Autodesk Inventor part; units mm, degrees
ref_plane "YZ Plane" through (0, 0, 0) normal (1, 0, 0) x (0, 1, 0)
ref_plane "XZ Plane" through (0, 0, 0) normal (0, 1, 0) x (-1, 0, 0)
ref_plane "XY Plane" through (0, 0, 0) normal (0, 0, 1) x (1, 0, 0)
sketch "Sketch1" plane through (0, 0, 0) normal (0, 1, 0) x (-1, 0, 0)
  line L0 (32, 32) -> (0, 32)
  line L1 (0, 32) -> (0, 0)
  line L2 (0, 0) -> (32, 0)
  line L3 (32, 0) -> (32, 32)
extrude "Extrusion1" add sketch "Sketch1" along normal blind 55
sketch "Sketch2" plane through (0, 55, 0) normal (0, 1, 0) x (1, 0, 0)
  line L0 (-9.6, -9.6) -> (-22.4, -9.6)
  line L1 (-22.4, -9.6) -> (-22.4, -22.4)
  line L2 (-22.4, -22.4) -> (-9.6, -22.4)
  line L3 (-9.6, -22.4) -> (-9.6, -9.6)
  point P0 (0, 0)
extrude "Extrusion2" cut sketch "Sketch2" against normal blind 30
sketch "Sketch3" plane through (-32, 0, 32) normal (0, 0, 1) x (1, 0, 0)
  line L0 (3.5, 49) -> (28.5, 49)
  line L1 (28.5, 49) -> (28.5, 31)
  line L2 (28.5, 31) -> (3.5, 31)
  line L3 (3.5, 31) -> (3.5, 49)
  line L4 (3.5, 49) -> (3.5, 43.25)
  line L5 (3.5, 36.75) -> (3.5, 43.25)
  line L6 (28.5, 49) -> (28.5, 43.25)
  line L7 (28.5, 36.75) -> (28.5, 43.25)
  line L8 (3.5, 43.25) -> (3.5, 36.75)
  line L9 (28.5, 43.25) -> (28.5, 36.75)
  point P0 (32, 0)
extrude "Extrusion3" cut sketch "Sketch3" against normal blind 2.5
sketch "Sketch4" plane through (-32, 0, 29.5) normal (0, 0, 1) x (1, 0, 0)
  line L0 (3.5, 49) -> (28.5, 49)
  line L1 (3.5, 49) -> (3.5, 43.25)
  line L2 (28.5, 31) -> (3.5, 31)
  line L3 (3.5, 36.75) -> (3.5, 31)
  line L4 (3.5, 31) -> (28.5, 31)
  line L5 (28.5, 31) -> (28.5, 36.75)
  line L6 (28.5, 49) -> (28.5, 31)
  line L7 (28.5, 43.25) -> (28.5, 49)
  line L8 (28.5, 49) -> (3.5, 49)
  point P0 (32, 0)
sketch "Sketch5" plane through (-32, 0, 29.5) normal (0, 0, 1) x (1, 0, 0)
  line L0 (3.5, 43.25) -> (8.5, 43.25)
  line L1 (8.5, 43.25) -> (8.5, 36.75)
  line L2 (8.5, 36.75) -> (3.5, 36.75)
  line L3 (3.5, 36.75) -> (3.5, 43.25)
  point P0 (32, 0)
sketch "Sketch6" plane through (-32, 0, 29.5) normal (0, 0, 1) x (1, 0, 0)
  line L0 (28.5, 43.25) -> (23.5, 43.25)
  line L1 (23.5, 43.25) -> (23.5, 36.75)
  line L2 (23.5, 36.75) -> (28.5, 36.75)
  line L3 (28.5, 36.75) -> (28.5, 43.25)
  point P0 (32, 0)
extrude "Extrusion4" cut sketch "Sketch5" against normal blind 2
extrude "Extrusion5" cut sketch "Sketch6" against normal blind 2
sketch "Sketch7" plane through (-32, 0, 29.5) normal (0, 0, 1) x (1, 0, 0)
  line L0 (3.5, 43.25) -> (8.5, 43.25)
  line L1 (3.5, 43.25) -> (3.5, 49)
  line L2 (8.5, 43.25) -> (3.5, 43.25)
  line L3 (3.5, 43.25) -> (3.5, 49)
  line L4 (3.5, 49) -> (8.5, 49)
  line L5 (8.5, 49) -> (8.5, 43.25)
  point P0 (32, 0)
sketch "Sketch8" plane through (-32, 0, 29.5) normal (0, 0, 1) x (1, 0, 0)
  line L0 (8.5, 36.75) -> (3.5, 36.75)
  line L1 (28.5, 31) -> (3.5, 31)
  line L2 (8.5, 36.75) -> (3.5, 36.75)
  line L3 (3.5, 36.75) -> (3.5, 31)
  line L4 (3.5, 31) -> (8.5, 31)
  line L5 (8.5, 31) -> (8.5, 36.75)
  point P0 (32, 0)
sketch "Sketch9" plane through (-32, 0, 29.5) normal (0, 0, 1) x (1, 0, 0)
  line L0 (28.5, 36.75) -> (23.5, 36.75)
  line L1 (28.5, 31) -> (3.5, 31)
  line L2 (23.5, 36.75) -> (28.5, 36.75)
  line L3 (28.5, 36.75) -> (28.5, 31)
  line L4 (28.5, 31) -> (23.5, 31)
  line L5 (23.5, 31) -> (23.5, 36.75)
  point P0 (32, 0)
sketch "Sketch10" plane through (-32, 0, 29.5) normal (0, 0, 1) x (1, 0, 0)
  line L0 (23.5, 43.25) -> (28.5, 43.25)
  line L1 (28.5, 49) -> (28.5, 43.25)
  line L2 (23.5, 43.25) -> (28.5, 43.25)
  line L3 (28.5, 43.25) -> (28.5, 49)
  line L4 (28.5, 49) -> (23.5, 49)
  line L5 (23.5, 49) -> (23.5, 43.25)
  point P0 (32, 0)
extrude "Extrusion6" add sketch "Sketch7" along normal blind 1
extrude "Extrusion7" add sketch "Sketch8" along normal blind 1
extrude "Extrusion8" add sketch "Sketch9" along normal blind 1
extrude "Extrusion9" add sketch "Sketch10" along normal blind 1
sketch "Sketch11" plane through (-32, 0, 30.5) normal (0, 0, 1) x (1, 0, 0)
  line L0 (23.5, 43.25) -> (28.5, 43.25)
  line L1 (23.5, 43.25) -> (25, 43.25)
  line L2 (25, 43.25) -> (25, 44.25)
  line L3 (25, 44.25) -> (23.5, 44.25)
  line L4 (23.5, 44.25) -> (23.5, 43.25)
  point P0 (32, 0)
extrude "Extrusion10" cut sketch "Sketch11" against normal blind 1
sketch "Sketch12" plane through (-32, 0, 29.5) normal (0, 0, 1) x (1, 0, 0)
  line L0 (8.5, 49) -> (8.5, 43.25)
  line L1 (23.5, 31) -> (8.5, 31)
  line L2 (23.5, 49) -> (23.5, 44.25)
  point P0 (32, 0)
sketch "Sketch13" plane through (-32, 0, 29.5) normal (0, 0, 1) x (1, 0, 0)
  point P0 (32, 0)
sketch "Sketch14" plane through (-32, 0, 29.5) normal (0, 0, 1) x (1, 0, 0)
  line L0 (23.5, 44.25) -> (23.5, 49)
  line L1 (23.5, 49) -> (17.5, 49)
  line L2 (14.5, 43) -> (17.5, 43)
  line L3 (17.5, 38) -> (18, 38)
  line L4 (18, 38) -> (18, 43)
  line L5 (18, 43) -> (14, 43)
  line L6 (14, 43) -> (14, 38)
  line L7 (14, 38) -> (14.5, 38)
  line L8 (14.5, 38) -> (14.5, 42)
  line L9 (3.5, 43.25) -> (8.5, 43.25)
  line L10 (14.5, 42) -> (14.5, 42.5)
  line L11 (14.5, 42.5) -> (17.5, 42.5)
  line L12 (17.5, 42.5) -> (17.5, 38)
  point P0 (32, 0)
extrude "Extrusion11" add sketch "Sketch14" along normal blind 1
sketch "Sketch15" plane through (-32, 0, 29.5) normal (0, 0, 1) x (1, 0, 0)
  line L0 (14.5, 42.5) -> (14.5, 38)
  line L1 (14.5, 42.5) -> (17.5, 42.5)
  line L2 (17.5, 42.5) -> (17.5, 39.5)
  line L3 (17.5, 39.5) -> (14.5, 39.5)
  line L4 (14.5, 39.5) -> (14.5, 42.5)
  point P0 (32, 0)
extrude "Extrusion12" cut sketch "Sketch15" against normal blind 7.1
sketch "Sketch16" plane through (-32, 0, 32) normal (0, 0, 1) x (1, 0, 0)
  point P0 (32, 0)
sketch "Sketch17" plane through (0, 0, 32) normal (1, 0, 0) x (0, 0, -1)
  line L0 (2, 46) -> (20, 46)
  line L1 (20, 46) -> (20, 8)
  line L2 (20, 8) -> (2, 8)
  line L3 (2, 8) -> (2, 46)
  point P0 (32, 0)
extrude "Extrusion13" cut sketch "Sketch17" against normal blind 1.5
sketch "Sketch18" plane through (-1.5, 0, 32) normal (1, 0, 0) x (0, 0, -1)
  line L0 (20, 38.5) -> (14, 38.5)
  line L1 (14, 38.5) -> (14, 46)
  line L2 (14, 46) -> (20, 46)
  line L3 (20, 46) -> (20, 38.5)
  point P0 (32, 0)
extrude "Extrusion14" cut sketch "Sketch18" against normal blind 8.1
sketch "Sketch19" plane through (0, 55, 0) normal (0, 1, 0) x (1, 0, 0)
  circle A0 centre (-16, -16) radius 10.5
  point P0 (0, 0)
sketch "Sketch20" plane through (0, 55, 0) normal (0, 1, 0) x (1, 0, 0)
  point P0 (0, 0)
extrude "Extrusion15" cut sketch "Sketch19" against normal blind 2
sketch "Sketch21" plane through (-32, 0, 0) normal (-1, 0, 0) x (0, 0, 1)
  line L0 (32, 0) -> (32, 55)
  line L1 (0, 0) -> (32, 0)
  line L2 (32, 0) -> (32, 55)
  line L3 (32, 55) -> (0, 55)
  line L4 (0, 55) -> (0, 0)
extrude "Extrusion16" add sketch "Sketch21" along normal blind 4
sketch "Sketch22" plane through (-36, 0, 0) normal (-1, 0, 0) x (0, 0, 1)
  line L0 (2, 3) -> (4, 3)
  line L1 (4, 3) -> (4, 52)
  line L2 (4, 52) -> (2, 52)
  line L3 (2, 52) -> (2, 3)
  line L4 (23, 3) -> (25, 3)
  line L5 (25, 3) -> (25, 52)
  line L6 (25, 52) -> (23, 52)
  line L7 (23, 52) -> (23, 3)
  point P0 (0, 0)
extrude "Extrusion17" cut sketch "Sketch22" against normal blind 11
properties part number "Cuvette Holder v2_3DPrint"
For this review, take the finished solid that the model builds, in its own axes (mm). A direction names the side the tool comes from. Give positions to 0.01 mm unless a question says otherwise; leave off trailing zeros. Loops run counter-clockwise (first coordinate to the right, second up) from the corner with the lowest first, then second, coordinate; pieces in that order, holes last. Notation, with made-up numbers: M 12.25,48.5 L 43.25,48.5 A29 ccw 43.25,71.5 Z; hole C 28.25,75 d4. An arc over 180 degrees is marked long. Put each result on its own line as item: value. Start each with the question number.
(1) Add section A-A, the plane z = 16. Write out the cut boundary in (x, y).
(2) The part is to be moulded in two halves that separate along X. For faces 4 (the flat face through (-18, 0, 16)), 5 (the flat face through (0, 27, 9)), 6 (the flat face through (-16, 49, 31)), say which applies: +X half, -X half, draft (parallel to the pull), parting line (faces both ways), or undercut.
(3) Add section D-D, the plane y = 10.5. Write out the cut boundary in (x, z), then the cut area to 3 significant figures.
(4) Add section B-B, the plane y = 28.5. Write out the cut boundary in (x, z), then the cut area to 3 significant figures.
(5) For pin 1 (1.5 mm diameter, centred on x = -16.5, z = 25.5, fed in from +Y); pin 2 (4 mm diameter, centred on x = -26, y = 39, fed in from +Z), all flat-tipped, find the tip position at first contact; note any pin that passes through.
(6) Add section C-C, the plane x = -16. Write out the cut boundary in (y, z), then the cut area to 3 significant figures.
(7) Machinability: for faces 1 (the flat face through (-31, 52, 24)), 2 (the flat face through (-26, 40, 27.5)), 3 (the flat face through (-9.6, 36, 16)), which of the approach directions +Z, -Z, +X, -X, +Y, -Y give a long, thin tool a straight path to every point of the face, cutting with its end or side? Answer none if there is none.
(8) Wall thickness on L1, parallel to Z at x = -34, y = 26; L2, parallel to Z at x = -16, y = 53.65; L3, parallel to Z at x = -21.5, y = 44.5: over which ranges is each line inside the solid? List them lowest first.
Result:
1. outline: M -36,0 L 0,0 L 0,8 L -1.5,8 L -1.5,38.5 L -9.6,38.5 L -9.6,25 L -22.4,25 L -22.4,53 L -26.5,53 L -26.5,55 L -36,55 Z; M -9.6,46 L 0,46 L 0,55 L -5.5,55 L -5.5,53 L -9.6,53 Z
2. face 4: draft
2. face 5: +X half
2. face 6: undercut
3. outline: M -36,0 L 0,0 L 0,12 L -1.5,12 L -1.5,30 L 0,30 L 0,32 L -36,32 L -36,25 L -25,25 L -25,23 L -36,23 L -36,4 L -25,4 L -25,2 L -36,2 Z
3. area: 1,080 mm^2
4. outline: M -36,0 L 0,0 L 0,12 L -1.5,12 L -1.5,30 L 0,30 L 0,32 L -36,32 L -36,25 L -25,25 L -25,23 L -36,23 L -36,4 L -25,4 L -25,2 L -36,2 Z; hole M -22.4,9.6 L -9.6,9.6 L -9.6,22.4 L -22.4,22.4 Z
4. area: 917 mm^2
5. pin 1: stops at y = 53
5. pin 2: stops at z = 27.5
6. outline: M 0,0 L 55,0 L 55,5.5 L 53,5.5 L 53,9.6 L 25,9.6 L 25,22.4 L 39.5,22.4 L 39.5,29.5 L 31,29.5 L 31,32 L 0,32 Z; M 42.5,22.4 L 53,22.4 L 53,26.5 L 55,26.5 L 55,32 L 49,32 L 49,29.5 L 43,29.5 L 43,30.5 L 42.5,30.5 Z
6. area: 1,290 mm^2
7. face 1: -X
7. face 2: +Z
7. face 3: +Y
8. L1: z = 0 to 2, 4 to 23, 25 to 32
8. L2: z = 0 to 5.5, 26.5 to 32
8. L3: z = 0 to 9.6, 22.4 to 29.5
